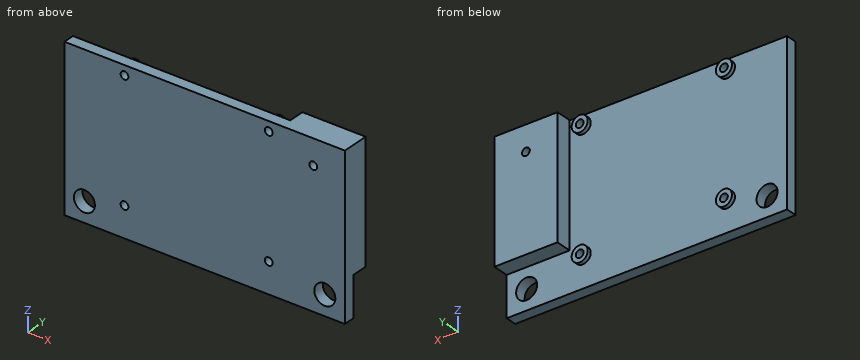
Autodesk Inventor part; units mm, degrees
ref_plane "YZ Plane" through (0, 0, 0) normal (1, 0, 0) x (0, 1, 0)
ref_plane "XZ Plane" through (0, 0, 0) normal (0, 1, 0) x (-1, 0, 0)
ref_plane "XY Plane" through (0, 0, 0) normal (0, 0, 1) x (1, 0, 0)
sketch "Sketch1" plane through (0, 0, 0) normal (0, 1, 0) x (-1, 0, 0)
  line L0 (49.0764, 56.1521) -> (-39.8236, 56.1521)
  line L1 (-39.8236, 56.1521) -> (-39.8236, 5.3521)
  line L2 (-39.8236, 5.3521) -> (49.0764, 5.3521)
  line L3 (49.0764, 5.3521) -> (49.0764, 56.1521)
  point P0 (0, 0)
  dimension "d0" = 88.9
  dimension "d1" = 50.8
extrude "Extrusion1" add sketch "Sketch1" along normal blind 3.556
sketch "Sketch2" plane through (0, 3.556, 0) normal (0, 1, 0) x (1, 0, 0)
  line L0 (39.8236, -56.1521) -> (39.8236, -5.3521)
  line L1 (39.8236, -5.3521) -> (-49.0764, -5.3521)
  point P0 (0, 0)
  point P1 (-42.7264, -11.7021)
  point P2 (33.4736, -11.7021)
  dimension "d4" = 76.2
  dimension "d5" = 0
  dimension "d6" = 6.35
  dimension "d7" = 6.35
hole "Hole1" at (-42.7264, 3.556, 11.7021) at (33.4736, 3.556, 11.7021) direction (0, -1, 0) diameter 6.6548 end through all
sketch "Sketch3" plane through (0, 3.556, 0) normal (0, 1, 0) x (1, 0, 0)
  circle A0 centre (-30.0264, -53.1041) radius 2.54
  circle A1 centre (-30.0264, -15.0041) radius 2.54
  line L0 (-49.0764, -56.1521) -> (39.8236, -56.1521)
  line L1 (-49.0764, -5.3521) -> (-49.0764, -56.1521)
  circle A2 centre (15.6936, -53.1041) radius 2.54
  circle A3 centre (15.6936, -15.0041) radius 2.54
  point P0 (0, 0)
  dimension "d15" = 5.08
  dimension "d16" = 5.08
  dimension "d17" = 3.048
  dimension "d18" = 38.1
  dimension "d19" = 0
  dimension "d20" = 19.05
  dimension "d21" = 5.08
  dimension "d22" = 0
  dimension "d23" = 45.72
  dimension "d24" = 5.08
  dimension "d25" = 0
  dimension "d26" = 0
extrude "Extrusion2" add sketch "Sketch3" along normal blind 1.27
sketch "Sketch4" plane through (-30.0264, 4.826, 15.0041) normal (0, 1, 0) x (1, 0, 0)
  circle A0 centre (0, 0) radius 2.54
  circle A1 centre (0, -38.1) radius 2.54
  circle A2 centre (45.72, -38.1) radius 2.54
  circle A3 centre (45.72, 0) radius 2.54
  circle A4 centre (45.72, 0) radius 2.54
  circle A5 centre (45.72, -38.1) radius 2.54
  point P0 (30.0264, 15.0041)
  point P1 (45.72, 0)
hole "Hole2" at (-30.0264, 4.826, 53.1041) at (-30.0264, 4.826, 15.0041) at (15.6936, 4.826, 15.0041) at (15.6936, 4.826, 53.1041) direction (0, -1, 0) diameter 2.4638 end through all
sketch "Sketch5" plane through (0, 3.556, 0) normal (0, 1, 0) x (1, 0, 0)
  line L0 (19.8236, -18.0521) -> (39.8236, -18.0521)
  line L1 (39.8236, -18.0521) -> (39.8236, -56.1521)
  line L2 (39.8236, -56.1521) -> (19.8236, -56.1521)
  line L3 (19.8236, -56.1521) -> (19.8236, -18.0521)
  line L4 (39.8236, -56.1521) -> (39.8236, -5.3521)
  line L5 (-49.0764, -56.1521) -> (39.8236, -56.1521)
  line L6 (39.8236, -5.3521) -> (-49.0764, -5.3521)
  point P0 (0, 0)
  dimension "d36" = 0
  dimension "d37" = 20
  dimension "d38" = 0
  dimension "d40" = 12.7
extrude "Extrusion3" add sketch "Sketch5" along normal blind 5.08
sketch "Sketch6" plane through (0, 8.636, 0) normal (0, 1, 0) x (1, 0, 0)
  line L0 (19.8236, -56.1521) -> (39.8236, -56.1521)
  line L1 (39.8236, -56.1521) -> (39.8236, -18.0521)
  point P0 (0, 0)
  point P1 (29.8236, -48.1521)
  dimension "d43" = 8
  dimension "d44" = 10
hole "Hole3" at (29.8236, 8.636, 48.1521) direction (0, -1, 0) diameter 2.4638 end through all
properties part number "SF GPS"
Can you work these out from the model? Positions are in its coordinate system, mm. Coordinates: 2 decimals unless noted, no trailing zeros. Order: outer loops, then holes, each group sorted by start corner. A loop starts at its lowest first (then second) coordinate and runs counter-clockwise, first axis right, second up. Notation, with made-up numbers: (84.5, 43.25) -> (122.5, 43.25) arc R19 cw to (122.5, 80.25) -> close; hole circle Ø2 at (34.25, 38.25). An arc over 180 degrees is marked (long way). Write each question's results on one line, items separated by ' | '.
Item 1: I want a section at B-B, the plane z = 22. Write out the boundary of the cut face in (x, y).
Results are:
outline: (-49.08, 0) -> (39.82, 0) -> (39.82, 8.64) -> (19.82, 8.64) -> (19.82, 3.56) -> (-49.08, 3.56) -> close
Item 2: I want a section at A-A, the plane z = 10. Write out the boundary of the cut face in (x, y), then the cut area to 3 significant figures.
Results are:
outline: (-49.08, 0) -> (-45.59, 0) -> (-45.59, 3.56) -> (-49.08, 3.56) -> close; (-39.87, 0) -> (30.61, 0) -> (30.61, 3.56) -> (-39.87, 3.56) -> close; (36.33, 0) -> (39.82, 0) -> (39.82, 3.56) -> (36.33, 3.56) -> close | area: 275 mm²
Item 3: I'm going to push flat-ended pins straight in: pin 1 Ø4 at (x, z) = (-31, 54) entering from +Y; pin 2 Ø3 at (x, z) = (-30.03, 53.1) entering from -Y; pin 3 Ø2.5 at (x, y) = (28, 7) entering from -Z; pin 4 Ø5 at (x, z) = (-12.5, 24) entering from +Y. Where does each tip first touch, or does it pass through?
Results are:
pin 1: y = 4.83 | pin 2: y = 0 | pin 3: z = 18.05 | pin 4: y = 3.56
Item 4: I want a section at C-C, the plane y = 2. Write out the boundary of the cut face in (x, z).
Results are:
outline: (-49.08, 5.35) -> (39.82, 5.35) -> (39.82, 56.15) -> (-49.08, 56.15) -> close; hole circle Ø6.65 at (-42.73, 11.7); hole circle Ø2.46 at (-30.03, 15); hole circle Ø2.46 at (-30.03, 53.1); hole circle Ø2.46 at (15.69, 15); hole circle Ø2.46 at (15.69, 53.1); hole circle Ø2.46 at (29.82, 48.15); hole circle Ø6.65 at (33.47, 11.7)
Item 5: If I drill on line 1 along X through (y, z) = (4.25, 22); line 2 along X through (y, z) = (4.75, 51); line 3 along Z through (x, y) = (27, 6.75), over which ranges is the centre line in solid material (lowest first)?
Results are:
line 1: 19.82 to 39.82 | line 2: -31.45 to -28.6, 14.27 to 17.12, 19.82 to 39.82 | line 3: 18.05 to 56.15
Item 6: I want a section at D-D, the plane x = -22.5. Write out the boundary of the cut face in (y, z), then the cut area to 3 significant figures.
Results are:
outline: (0, 5.35) -> (3.56, 5.35) -> (3.56, 56.15) -> (0, 56.15) -> close | area: 181 mm²
